The drawing under review shows one solid part. Ordinate dimensions are in mm from its lowest x, y, z. Coordinates: 2 decimals unless noted, no trailing zeros. Order: outer loops, then holes, each group sorted by start corner. A loop starts at its lowest first (then second) coordinate and runs counter-clockwise, first axis right, second up. Notation, with made-up numbers: M 12.25,62.25 L 24.25,62.25 A29 ccw 24.25,95.25 Z; hole C -19.75,63 d7. An arc over 180 degrees is marked long. Answer as a JSON object with one key per item and string values.
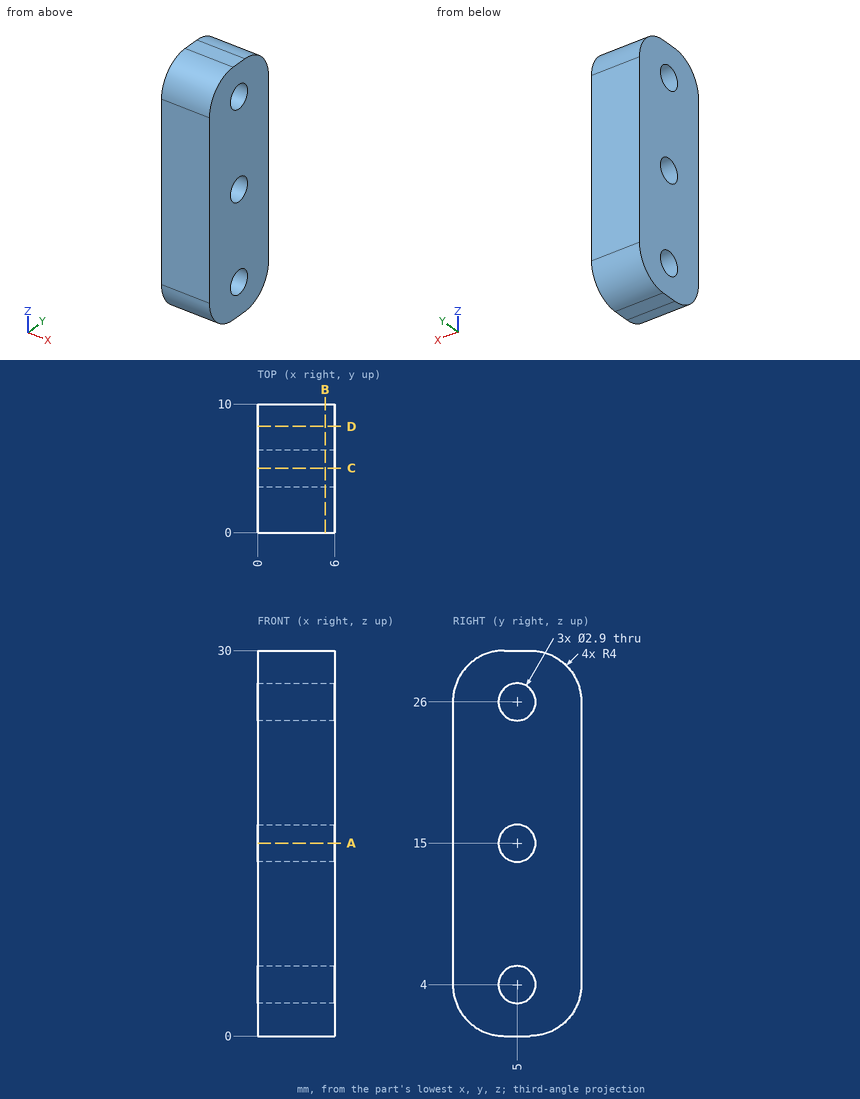
1) Add section A-A (z = 15). State the section outline as (x, y) points.
Taken from the geometry:
{"outline": "M 0,0 L 6,0 L 6,3.55 L 0,3.55 Z; M 0,6.45 L 6,6.45 L 6,10 L 0,10 Z"}
2) Add section D-D (y = 8.25). State the section outline as (x, z) points.
Taken from the geometry:
{"outline": "M 0,0.69 L 6,0.69 L 6,29.31 L 0,29.31 Z"}
3) To check wall thickness, follow L1, parallel to Y at x = 4.1, z = 4; L2, parallel to Z at x = 1.05, y = 3.75; L3, parallel to Z at x = 2.65, y = 4.5. State the ranges of each line that lie inside material, in increasing order.
Taken from the geometry:
{"L1": "y = 0 to 3.55, 6.45 to 10", "L2": "z = 0.01 to 3.27, 4.73 to 14.27, 15.73 to 25.27, 26.73 to 29.99", "L3": "z = 0 to 2.64, 5.36 to 13.64, 16.36 to 24.64, 27.36 to 30"}
4) Add section B-B (x = 5.25). State the section outline as (y, z) points.
Taken from the geometry:
{"outline": "M 0,4 A4 ccw 4,0 L 6,0 A4 ccw 10,4 L 10,26 A4 ccw 6,30 L 4,30 A4 ccw 0,26 Z; hole C 5,4 d2.9; hole C 5,15 d2.9; hole C 5,26 d2.9"}
5) Add section C-C (y = 5). State the section outline as (x, z) points, and give its area (3 significant figures).
Taken from the geometry:
{"outline": "M 0,0 L 6,0 L 6,2.55 L 0,2.55 Z; M 0,5.45 L 6,5.45 L 6,13.55 L 0,13.55 Z; M 0,16.45 L 6,16.45 L 6,24.55 L 0,24.55 Z; M 0,27.45 L 6,27.45 L 6,30 L 0,30 Z", "area": "128 mm2"}
